Could you check a few things on this model? Use its own coordinates, in mm. A direction names the side the tool comes from. Round coordinates to 2 decimals unless told otherwise and drop trailing zeros. Order: outer loops, then holes, each group sorted by start corner. A loop starts at its lowest first (then second) coordinate and runs counter-clockwise, first axis right, second up. Notation, with made-up numbers: (-15.75, 55.5) - (15.25, 55.5) arc R24 ccw to (15.25, 86.5) - close; hole circle Ø1 at (7.5, 71.5). An arc over 180 degrees is marked (long way). Use one line per item in the form item = value.
from build123d import *

# Parameters (mm, degrees)
SKETCH1_W               = 14
SKETCH1_H               = 24
SKETCH1_W_2             = 3
SKETCH1_H_2             = 3
PCB_DEPTH               = 1.2
SOLDER_JOINTS_DEPTH     = 1
SOLDER_FILLETS_R        = 1.125
SKETCH2_W               = 3.205722041
SKETCH2_H               = 3.205722042
SKETCH2_W_2             = 3.205722042
SKETCH2_W_3             = 2.430144128
SKETCH2_H_2             = 4.007152552
TOP_COMPONENTS_DEPTH    = 1
SKETCH3_W               = 4.033005149
SKETCH3_H               = 4.058308378
SKETCH3_W_2             = 3.102311653
SKETCH3_H_2             = 2.921343474
SKETCH3_W_3             = 2.817933085
SKETCH3_W_4             = 2.869638279
SKETCH3_W_5             = 1.835534395
SKETCH3_H_3             = 3.12816425
BOTTOM_COMPONENTS_DEPTH = 1


with BuildPart() as part:
    # Sketch1 → PCB (new body)
    with BuildSketch(Plane(origin=(0, 0, 0), x_dir=(1, 0, 0), z_dir=(0, 1, 0))):
        Rectangle(SKETCH1_W, SKETCH1_H)
        with Locations((-5.5, 13.5)):
            Rectangle(SKETCH1_W_2, SKETCH1_H_2)
        with Locations((0, 13.5)):
            Rectangle(SKETCH1_W_2, SKETCH1_H_2)
        with Locations((5.5, 13.5)):
            Rectangle(SKETCH1_W_2, SKETCH1_H_2)
    extrude(amount=PCB_DEPTH)

    # Sketch5 → Solder joints (add)
    with BuildSketch(Plane(origin=(0, 1.2, 0), x_dir=(1, 0, 0), z_dir=(0, 1, 0))):
        with BuildLine():
            Line((-4.375, 13.25), (-4.375, 13.75))
            ThreePointArc((-4.375, 13.75), (-5.5, 14.875), (-6.625, 13.75))
            Line((-6.625, 13.75), (-6.625, 13.25))
            ThreePointArc((-6.625, 13.25), (-5.5, 12.125), (-4.375, 13.25))
        make_face()
        with BuildLine():
            Line((-1.125, 13.75), (-1.125, 13.25))
            ThreePointArc((-1.125, 13.25), (0, 12.125), (1.125, 13.25))
            Line((1.125, 13.25), (1.125, 13.75))
            ThreePointArc((1.125, 13.75), (0, 14.875), (-1.125, 13.75))
        make_face()
        with BuildLine():
            Line((4.375, 13.75), (4.375, 13.25))
            ThreePointArc((4.375, 13.25), (5.5, 12.125), (6.625, 13.25))
            Line((6.625, 13.25), (6.625, 13.75))
            ThreePointArc((6.625, 13.75), (5.5, 14.875), (4.375, 13.75))
        make_face()
        with BuildLine():
            Line((-6.625, -10.25), (-6.625, -10.75))
            ThreePointArc((-6.625, -10.75), (-5.5, -11.875), (-4.375, -10.75))
            Line((-4.375, -10.75), (-4.375, -10.25))
            ThreePointArc((-4.375, -10.25), (-5.5, -9.125), (-6.625, -10.25))
        make_face()
        with BuildLine():
            ThreePointArc((6.625, -10.75), (5.5, -11.875), (4.375, -10.75))
            Line((4.375, -10.75), (4.375, -10.25))
            ThreePointArc((4.375, -10.25), (5.5, -9.125), (6.625, -10.25))
            Line((6.625, -10.25), (6.625, -10.75))
        make_face()
    extrude(amount=SOLDER_JOINTS_DEPTH)

    # Solder fillets
    # the kernel refuses this fillet: 1.125 mm, written as the material it takes off along each edge
    with BuildSketch(Plane(origin=(-5.5, 2.2, 10.25), x_dir=(1, 0, 0), z_dir=(0, 0, 1))) as solder_fillets_piece_1:
        with BuildLine():
            CenterArc((0.006966011, -1.125), SOLDER_FILLETS_R, 6.379370208, 83.620629792)
            Line((0.006966011, 0), (0.006966011, 0.0225))
            Line((0.006966011, 0.0225), (1.125, 0.0225))
            Line((1.125, 0.0225), (1.1475, 0))
            ThreePointArc((1.1475, 0), (1.1475, -0.5), (1.14736068, -0.9975))
            Line((1.14736068, -0.9975), (1.125, -1))
        make_face()
    revolve(axis=Axis((-5.5, 2.2, 10.25), (0, 1, 0)), revolution_arc=180, mode=Mode.SUBTRACT)
    with BuildSketch(Plane(origin=(-4.375, 2.2, 10.75), x_dir=(0, -1, 0), z_dir=(0, 0, -1)), Plane(origin=(-6.625, 2.2, 10.25), x_dir=(0, -1, 0), z_dir=(0, 0, 1)), Plane(origin=(6.625, 2.2, -13.25), x_dir=(0, -1, 0), z_dir=(0, 0, -1)), Plane(origin=(4.375, 2.2, -13.75), x_dir=(0, -1, 0), z_dir=(0, 0, 1)), Plane(origin=(1.125, 2.2, -13.25), x_dir=(0, -1, 0), z_dir=(0, 0, -1)), Plane(origin=(-1.125, 2.2, -13.75), x_dir=(0, -1, 0), z_dir=(0, 0, 1)), Plane(origin=(-6.625, 2.2, -13.75), x_dir=(0, -1, 0), z_dir=(0, 0, 1)), Plane(origin=(-4.375, 2.2, -13.25), x_dir=(0, -1, 0), z_dir=(0, 0, -1))) as solder_fillets_piece_2:
        with BuildLine():
            CenterArc((1.125, 1.118033989), SOLDER_FILLETS_R, 180, 83.620629792)
            Line((0, 1.118033989), (-0.0225, 1.118033989))
            Line((-0.0225, 1.118033989), (-0.0225, 0))
            Line((-0.0225, 0), (0, -0.0225))
            ThreePointArc((0, -0.0225), (0.5, -0.0225), (0.9975, -0.02236068))
            Line((0.9975, -0.02236068), (1, 0))
        make_face()
    extrude(amount=0.5, mode=Mode.SUBTRACT)
    with BuildSketch(Plane(origin=(-5.5, 2.2, 10.75), x_dir=(-1, 0, 0), z_dir=(0, 0, -1))) as solder_fillets_piece_3:
        with BuildLine():
            CenterArc((0.006966011, -1.125), SOLDER_FILLETS_R, 6.379370208, 83.620629792)
            Line((0.006966011, 0), (0.006966011, 0.0225))
            Line((0.006966011, 0.0225), (1.125, 0.0225))
            Line((1.125, 0.0225), (1.1475, 0))
            ThreePointArc((1.1475, 0), (1.1475, -0.5), (1.14736068, -0.9975))
            Line((1.14736068, -0.9975), (1.125, -1))
        make_face()
    revolve(axis=Axis((-5.5, 2.2, 10.75), (0, 1, 0)), revolution_arc=180, mode=Mode.SUBTRACT)
    with BuildSketch(Plane(origin=(4.375, 2.2, 10.75), x_dir=(0, -1, 0), z_dir=(0, 0, -1)), Plane(origin=(6.625, 2.2, 10.25), x_dir=(0, -1, 0), z_dir=(0, 0, 1))) as solder_fillets_piece_4:
        with BuildLine():
            CenterArc((1.125, -1.118033989), SOLDER_FILLETS_R, 96.379370208, 83.620629792)
            Line((0, -1.118033989), (-0.0225, -1.118033989))
            Line((-0.0225, -1.118033989), (-0.0225, 0))
            Line((-0.0225, 0), (0, 0.0225))
            ThreePointArc((0, 0.0225), (0.5, 0.0225), (0.9975, 0.02236068))
            Line((0.9975, 0.02236068), (1, 0))
        make_face()
    extrude(amount=0.5, mode=Mode.SUBTRACT)
    with BuildSketch(Plane(origin=(5.5, 2.2, 10.25), x_dir=(-1, 0, 0), z_dir=(0, 0, 1))) as solder_fillets_piece_5:
        with BuildLine():
            CenterArc((0.006966011, 1.125), SOLDER_FILLETS_R, 270, 83.620629792)
            Line((0.006966011, 0), (0.006966011, -0.0225))
            Line((0.006966011, -0.0225), (1.125, -0.0225))
            Line((1.125, -0.0225), (1.1475, 0))
            ThreePointArc((1.1475, 0), (1.1475, 0.5), (1.14736068, 0.9975))
            Line((1.14736068, 0.9975), (1.125, 1))
        make_face()
    revolve(axis=Axis((5.5, 2.2, 10.25), (0, -1, 0)), revolution_arc=180, mode=Mode.SUBTRACT)
    with BuildSketch(Plane(origin=(5.5, 2.2, 10.75), x_dir=(1, 0, 0), z_dir=(0, 0, -1))) as solder_fillets_piece_6:
        with BuildLine():
            CenterArc((0.006966011, 1.125), SOLDER_FILLETS_R, 270, 83.620629792)
            Line((0.006966011, 0), (0.006966011, -0.0225))
            Line((0.006966011, -0.0225), (1.125, -0.0225))
            Line((1.125, -0.0225), (1.1475, 0))
            ThreePointArc((1.1475, 0), (1.1475, 0.5), (1.14736068, 0.9975))
            Line((1.14736068, 0.9975), (1.125, 1))
        make_face()
    revolve(axis=Axis((5.5, 2.2, 10.75), (0, -1, 0)), revolution_arc=180, mode=Mode.SUBTRACT)
    with BuildSketch(Plane(origin=(5.5, 2.2, -13.75), x_dir=(1, 0, 0), z_dir=(0, 0, 1))) as solder_fillets_piece_7:
        with BuildLine():
            CenterArc((0.006966011, -1.125), SOLDER_FILLETS_R, 6.379370208, 83.620629792)
            Line((0.006966011, 0), (0.006966011, 0.0225))
            Line((0.006966011, 0.0225), (1.125, 0.0225))
            Line((1.125, 0.0225), (1.1475, 0))
            ThreePointArc((1.1475, 0), (1.1475, -0.5), (1.14736068, -0.9975))
            Line((1.14736068, -0.9975), (1.125, -1))
        make_face()
    revolve(axis=Axis((5.5, 2.2, -13.75), (0, 1, 0)), revolution_arc=180, mode=Mode.SUBTRACT)
    with BuildSketch(Plane(origin=(5.5, 2.2, -13.25), x_dir=(-1, 0, 0), z_dir=(0, 0, -1))) as solder_fillets_piece_8:
        with BuildLine():
            CenterArc((0.006966011, -1.125), SOLDER_FILLETS_R, 6.379370208, 83.620629792)
            Line((0.006966011, 0), (0.006966011, 0.0225))
            Line((0.006966011, 0.0225), (1.125, 0.0225))
            Line((1.125, 0.0225), (1.1475, 0))
            ThreePointArc((1.1475, 0), (1.1475, -0.5), (1.14736068, -0.9975))
            Line((1.14736068, -0.9975), (1.125, -1))
        make_face()
    revolve(axis=Axis((5.5, 2.2, -13.25), (0, 1, 0)), revolution_arc=180, mode=Mode.SUBTRACT)
    with BuildSketch(Plane(origin=(0, 2.2, -13.75), x_dir=(1, 0, 0), z_dir=(0, 0, 1))) as solder_fillets_piece_9:
        with BuildLine():
            CenterArc((0.006966011, -1.125), SOLDER_FILLETS_R, 6.379370208, 83.620629792)
            Line((0.006966011, 0), (0.006966011, 0.0225))
            Line((0.006966011, 0.0225), (1.125, 0.0225))
            Line((1.125, 0.0225), (1.1475, 0))
            ThreePointArc((1.1475, 0), (1.1475, -0.5), (1.14736068, -0.9975))
            Line((1.14736068, -0.9975), (1.125, -1))
        make_face()
    revolve(axis=Axis((0, 2.2, -13.75), (0, 1, 0)), revolution_arc=180, mode=Mode.SUBTRACT)
    with BuildSketch(Plane(origin=(0, 2.2, -13.25), x_dir=(-1, 0, 0), z_dir=(0, 0, -1))) as solder_fillets_piece_10:
        with BuildLine():
            CenterArc((0.006966011, -1.125), SOLDER_FILLETS_R, 6.379370208, 83.620629792)
            Line((0.006966011, 0), (0.006966011, 0.0225))
            Line((0.006966011, 0.0225), (1.125, 0.0225))
            Line((1.125, 0.0225), (1.1475, 0))
            ThreePointArc((1.1475, 0), (1.1475, -0.5), (1.14736068, -0.9975))
            Line((1.14736068, -0.9975), (1.125, -1))
        make_face()
    revolve(axis=Axis((0, 2.2, -13.25), (0, 1, 0)), revolution_arc=180, mode=Mode.SUBTRACT)
    with BuildSketch(Plane(origin=(-5.5, 2.2, -13.25), x_dir=(-1, 0, 0), z_dir=(0, 0, -1))) as solder_fillets_piece_11:
        with BuildLine():
            CenterArc((0.006966011, -1.125), SOLDER_FILLETS_R, 6.379370208, 83.620629792)
            Line((0.006966011, 0), (0.006966011, 0.0225))
            Line((0.006966011, 0.0225), (1.125, 0.0225))
            Line((1.125, 0.0225), (1.1475, 0))
            ThreePointArc((1.1475, 0), (1.1475, -0.5), (1.14736068, -0.9975))
            Line((1.14736068, -0.9975), (1.125, -1))
        make_face()
    revolve(axis=Axis((-5.5, 2.2, -13.25), (0, 1, 0)), revolution_arc=180, mode=Mode.SUBTRACT)
    with BuildSketch(Plane(origin=(-5.5, 2.2, -13.75), x_dir=(1, 0, 0), z_dir=(0, 0, 1))) as solder_fillets_piece_12:
        with BuildLine():
            CenterArc((0.006966011, -1.125), SOLDER_FILLETS_R, 6.379370208, 83.620629792)
            Line((0.006966011, 0), (0.006966011, 0.0225))
            Line((0.006966011, 0.0225), (1.125, 0.0225))
            Line((1.125, 0.0225), (1.1475, 0))
            ThreePointArc((1.1475, 0), (1.1475, -0.5), (1.14736068, -0.9975))
            Line((1.14736068, -0.9975), (1.125, -1))
        make_face()
    revolve(axis=Axis((-5.5, 2.2, -13.75), (0, 1, 0)), revolution_arc=180, mode=Mode.SUBTRACT)

    # Sketch2 → Top components (add)
    with BuildSketch(Plane(origin=(0, 1.2, 0), x_dir=(1, 0, 0), z_dir=(0, 1, 0))):
        with Locations((-4.369088912, 8.144117457)):
            Rectangle(SKETCH2_W, SKETCH2_H)
        with Locations((0.232673374, 8.144117457)):
            Rectangle(SKETCH2_W_2, SKETCH2_H)
        with Locations((4.860288257, 8.144117457)):
            Rectangle(SKETCH2_W, SKETCH2_H)
        with Locations((-4.937846048, 1.758525971)):
            Rectangle(SKETCH2_W_2, SKETCH2_H)
        with Locations((-0.18096818, 1.758525971)):
            Rectangle(SKETCH2_W_2, SKETCH2_H)
        with Locations((4.524204494, 1.758525971)):
            Rectangle(SKETCH2_W_2, SKETCH2_H)
        with Locations((-2.119912963, -3.68344572)):
            Rectangle(SKETCH2_W_3, SKETCH2_H_2)
    extrude(amount=TOP_COMPONENTS_DEPTH)

    # Sketch3 → Bottom components (add)
    with BuildSketch(Plane.XZ):
        with Locations((-0.775577914, 2.029154189)):
            Rectangle(SKETCH3_W, SKETCH3_H)
        with Locations((-4.343236315, -5.442521059)):
            Rectangle(SKETCH3_W_2, SKETCH3_H_2)
        with Locations((0.090484089, -5.442521059)):
            Rectangle(SKETCH3_W_3, SKETCH3_H_2)
        with Locations((4.511278196, -5.442521059)):
            Rectangle(SKETCH3_W_4, SKETCH3_H_2)
        with Locations((4.433720405, 7.923271646)):
            Rectangle(SKETCH3_W_5, SKETCH3_H_3)
    extrude(amount=BOTTOM_COMPONENTS_DEPTH)


solid = part.part
Item 1: Imagine slicing it at B-B on x = -2.5. Please give me the cut outline in (y, z).
Found:
outline = (-1, 0) - (0, 0) - (0, -12) - (1.2, -12) - (1.2, 1.68) - (2.2, 1.68) - (2.2, 5.69) - (1.2, 5.69) - (1.2, 12) - (0, 12) - (0, 4.06) - (-1, 4.06) - close
Item 2: Imagine slicing it at D-D on z = -4.25. Please give me the cut outline in (x, y), plus the area to 3 significant figures.
Found:
outline = (-7, 0) - (-5.89, 0) - (-5.89, -1) - (-2.79, -1) - (-2.79, 0) - (-1.32, 0) - (-1.32, -1) - (1.5, -1) - (1.5, 0) - (3.08, 0) - (3.08, -1) - (5.95, -1) - (5.95, 0) - (7, 0) - (7, 1.2) - (-7, 1.2) - close
area = 25.6 mm2
Item 3: Imagine slicing it at C-C on z = 7.75. Please give me the cut outline in (x, y), plus the area to 3 significant figures.
Found:
outline = (-7, 0) - (3.52, 0) - (3.52, -1) - (5.35, -1) - (5.35, 0) - (7, 0) - (7, 1.2) - (-7, 1.2) - close
area = 18.6 mm2
Item 4: Will these pins go through, and if not, where does the flat tip stop? P1, Ø0.5, axis at y = -0.5, z = -5, coming from the +X side; P2, Ø0.5, axis at y = 1.5, z = -1.5, coming from the +X side; P3, Ø0.6, axis at x = 3, y = 1, coming from the -Z side.
Found:
P1 = 5.95
P2 = 6.13
P3 = -12
Item 5: For faces 4 (the face through (6.265, 1.906, 10.496)), 5 (the face through (3, 1, -12)), 6 (the face through (0, 2, -3.361)), which set-ups out of +Z, -Z, +X, -X, +Y, -Y let a thin tool reach every point of the face, with its end or its side?
Found:
face_4 = +Z, +X, +Y
face_5 = -Z, +Y, -Y
face_6 = +X, -X, +Y
Item 6: I need wall thicknesses on L1, parallel to Z at x = 0, y = 2; L2, parallel to Z at x = -1, y = -0.55; L3, parallel to Z at x = 5.25, y = 1.9. Which ranges of each line are inside material? Lowest first, please.
Found:
L1 = -14.4 to -12.6, -9.75 to -6.54, -3.36 to -0.16
L2 = -6.9 to -3.98, 0 to 4.06
L3 = -14.48 to -12.52, -9.75 to -6.54, -3.36 to -0.16, 9.52 to 11.48
Item 7: Imagine slicing it at A-A on y = -0.3. Please give me the cut outline in (x, z).
Found:
outline = (-5.89, -6.9) - (-2.79, -6.9) - (-2.79, -3.98) - (-5.89, -3.98) - close; (-2.79, 0) - (1.24, 0) - (1.24, 4.06) - (-2.79, 4.06) - close; (-1.32, -6.9) - (1.5, -6.9) - (1.5, -3.98) - (-1.32, -3.98) - close; (3.08, -6.9) - (5.95, -6.9) - (5.95, -3.98) - (3.08, -3.98) - close; (3.52, 6.36) - (5.35, 6.36) - (5.35, 9.49) - (3.52, 9.49) - close
Item 8: If we mould it in two halves opening along X, with no side actions, what happens to faces 1 (the face through (0, 2.2, -8)), 2 (the face through (-0.905, 2, 4)), 3 (the face through (0, 1.2, 1))? For each: released by +X, released by -X, zero draft, split by the parting line, or undercut.
Found:
face_1 = zero draft
face_2 = released by +X
face_3 = undercut
